For this review, use the dimensioned drawing (mm, ordinates from the lowest corner) and the shaded views. Give positions to 0.01 mm unless a question says otherwise; leave off trailing zeros. Order: outer loops, then holes, each group sorted by start corner. A loop starts at its lowest first (then second) coordinate and runs counter-clockwise, first axis right, second up.
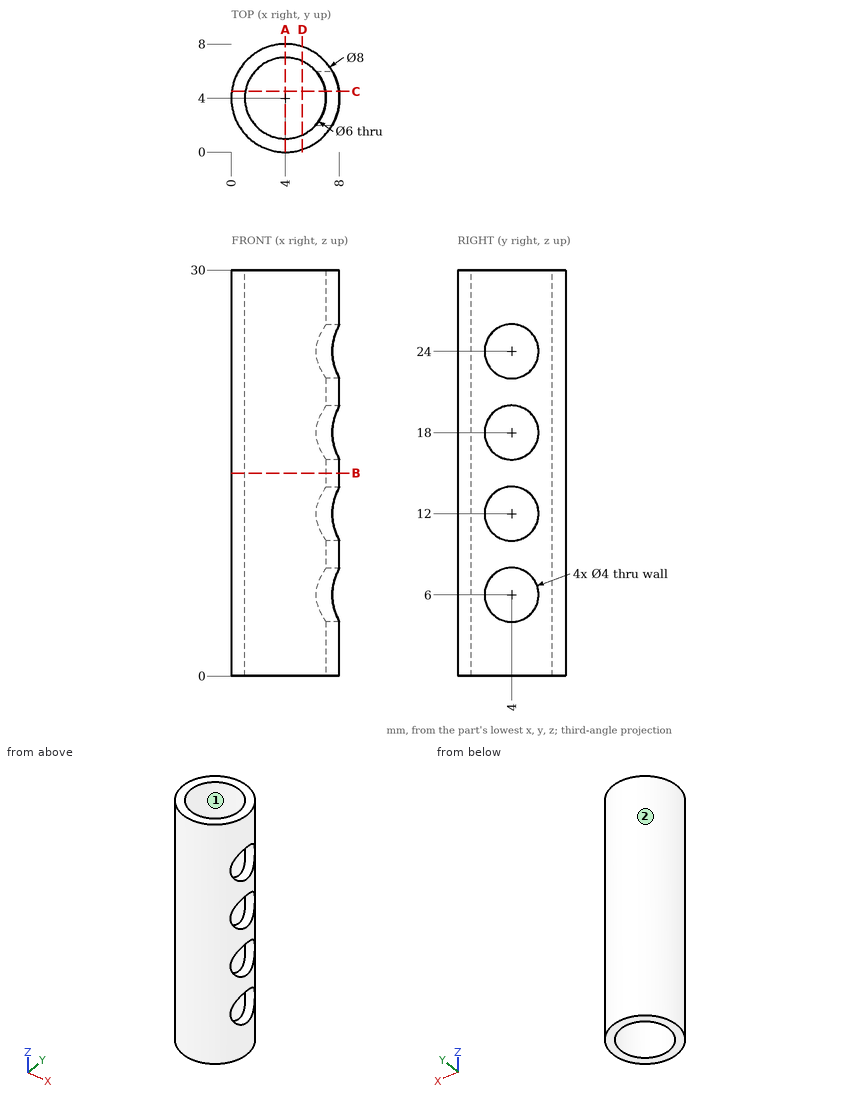
1. Take a section at D-D (x = 5.25). State the section outline as (y, z) points, then the cut area to 3 significant figures.
Recorded:
outline: (0.2, 0) - (1.27, 0) - (1.27, 30) - (0.2, 30) - close; (6.73, 0) - (7.8, 0) - (7.8, 30) - (6.73, 30) - close
area: 64.3 mm2
2. Take a section at A-A (x = 4). State the section outline as (y, z) points, then the cut area to 3 significant figures.
Recorded:
outline: (0, 0) - (1, 0) - (1, 30) - (0, 30) - close; (7, 0) - (8, 0) - (8, 30) - (7, 30) - close
area: 60.0 mm2
3. For line 1 along Y through (x, z) = (4, 24); line 2 along X through (y, z) = (6, 15); line 3 along Y through (x, z) = (6.65, 12), list the stretches that pass through material, from the lowest coordinate up.
Recorded:
line 1: y = 0 to 1, 7 to 8
line 2: x = 0.54 to 1.76, 6.24 to 7.46
line 3: y = 1 to 2, 6 to 7
4. Take a section at C-C (y = 4.5). State the section outline as (x, z) points.
Recorded:
outline: (0.03, 0) - (1.04, 0) - (1.04, 30) - (0.03, 30) - close; (6.96, 0) - (7.97, 0) - (7.97, 4.06) - (6.96, 4.06) - close; (6.96, 7.94) - (7.97, 7.94) - (7.97, 10.06) - (6.96, 10.06) - close; (6.96, 13.94) - (7.97, 13.94) - (7.97, 16.06) - (6.96, 16.06) - close; (6.96, 19.94) - (7.97, 19.94) - (7.97, 22.06) - (6.96, 22.06) - close; (6.96, 25.94) - (7.97, 25.94) - (7.97, 30) - (6.96, 30) - close
5. Draft analysis for pull direction X (two halves, no side actions). For the marked faces 1 and 2, state which applies: pulls with the +X half, pulls with the -X half, needs draft (parallel to the pull), parting line crosses it, or undercut.
Recorded:
face 1: undercut
face 2: parting line crosses it
6. Take a section at B-B (z = 15). State the section outline as (x, y) points, then the cut area to 3 significant figures.
Recorded:
outline: circle Ø8 at (4, 4); hole circle Ø6 at (4, 4)
area: 22.0 mm2
7. For pin 1 (1 mm diameter, centred on x = 3, z = 5, fed in from +Y); pin 2 (2.5 mm diameter, centred on y = 4, z = 18, fed in from +X), all flat-tipped, find the tip position at first contact; note any pin that passes through.
Recorded:
pin 1: stops at y = 7.97
pin 2: stops at x = 1.27
